from build123d import *

# Parameters (mm, degrees)
SKETCH1_R           = 0.3
SKETCH1_R_2         = 0.6
BOSS_EXTRUDE1_DEPTH = 5


with BuildPart() as part:
    # Sketch1 → Boss-Extrude1 (new body)
    with BuildSketch(Plane(origin=(0, 0, 0), x_dir=(1, 0, 0), z_dir=(0, 1, 0))):
        with BuildLine():
            ThreePointArc((0.1641009, 1.993256355), (0.024548565, 1.994973575), (-0.113883759, 1.977245221))
            Line((-0.113883759, 1.977245221), (-1.25, 1.750241174))
            Line((-1.25, 1.750241174), (-4.183235691, 1.164159973))
            ThreePointArc((-4.183235691, 1.164159973), (-4.514100231, 1.033532975), (-4.77830642, 0.795352694))
            ThreePointArc((-4.77830642, 0.795352694), (-5.05, 0), (-4.77830642, -0.795352694))
            ThreePointArc((-4.77830642, -0.795352694), (-4.514100231, -1.033532975), (-4.183235691, -1.164159973))
            Line((-4.183235691, -1.164159973), (-1.25, -1.750241174))
            Line((-1.25, -1.750241174), (-0.11388376, -1.977245221))
            ThreePointArc((-0.11388376, -1.977245221), (0.024548564, -1.994973575), (0.164100898, -1.993256355))
            ThreePointArc((0.164100898, -1.993256355), (2, -1e-09), (0.1641009, 1.993256355))
        make_face()
        with Locations(Location((-3, 0, 0), (0, 0, 270))):
            Circle(SKETCH1_R, mode=Mode.SUBTRACT)
        with Locations(Location((-1.25, 0, 0), (0, 0, 270))):
            Circle(SKETCH1_R_2, mode=Mode.SUBTRACT)
        with Locations(Location((0.5, 0, 0), (0, 0, 270))):
            Circle(SKETCH1_R, mode=Mode.SUBTRACT)
    extrude(amount=BOSS_EXTRUDE1_DEPTH)


solid = part.part
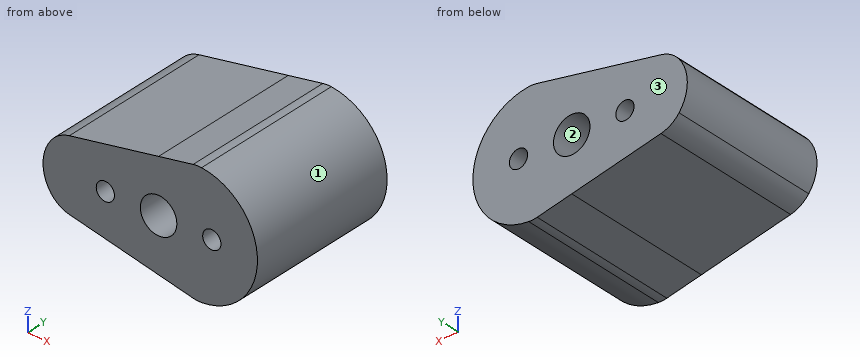
Geometry check sheet. Reference: the model listing, model coordinates, mm. Face numbers are marked on the shaded views. Coordinates: 2 decimals unless noted, no trailing zeros. Order: outer loops, then holes, each group sorted by start corner. A loop starts at its lowest first (then second) coordinate and runs counter-clockwise, first axis right, second up. Notation, with made-up numbers: (84.25, 21) -> (111.25, 21) arc R12 cw to (111.25, 43) -> close; hole circle Ø2 at (87.5, 65.5). An arc over 180 degrees is marked (long way). Use a Markdown table: item, result. Add a question column.
1. Cross-section at A-A (z = 0). Enter the section's corners in (x, y), and give its area (4 significant figures).
2. Material ranges on L1, parallel to Z at x = 0, y = 2.3; L2, parallel to X at y = 0.4, z = -0.35; L3, parallel to Z at x = -2, y = 0.8, recorded low to high.
3. Mould release check, pull along Z, two halves, no side actions. Record for the marked faces 1, 2 and 3: pulls with the +Z half, pulls with the -Z half, needs draft (parallel to the pull), parting line crosses it, or undercut.
4. Cross-section at B-B (x = -3). Enter the section's corners in (y, z).
5. Cross-section at C-C (y = 2.85). Enter the section's corners in (x, z).
6. Go/stop test with a flat-tipped pin: pin 1 Ø2 at (y, z) = (0.5, 1.5) entering from -X. Record where the tip stops, or that it passes through.
7. Cross-section at D-D (z = 0.5). Enter the section's corners in (x, y), and give its area (3 significant figures).
Filled sheet:
| question | item | result |
|---|---|---|
| 1 | outline | (-5.05, 0) -> (-3.3, 0) -> (-3.3, 5) -> (-5.05, 5) -> close; (-2.7, 0) -> (-1.85, 0) -> (-1.85, 5) -> (-2.7, 5) -> close; (-0.65, 0) -> (0.2, 0) -> (0.2, 5) -> (-0.65, 5) -> close; (0.8, 0) -> (2, 0) -> (2, 5) -> (0.8, 5) -> close |
| 1 | area | 23.25 mm2 |
| 2 | L1 | -1.99 to 1.99 |
| 2 | L2 | -5 to -1.74, -0.76 to 1.97 |
| 2 | L3 | -1.6 to 1.6 |
| 3 | face 1 | parting line crosses it |
| 3 | face 2 | undercut |
| 3 | face 3 | needs draft |
| 4 | outline | (0, -1.4) -> (5, -1.4) -> (5, -0.3) -> (0, -0.3) -> close; (0, 0.3) -> (5, 0.3) -> (5, 1.4) -> (0, 1.4) -> close |
| 5 | outline | (-4.78, -0.8) arc R1 ccw to (-4.18, -1.16) -> (-0.11, -1.98) arc R1 ccw to (0.16, -1.99) arc R2 ccw to (0.16, 1.99) arc R1 ccw to (-0.11, 1.98) -> (-4.18, 1.16) arc R1 ccw to (-4.78, 0.8) arc R1.3 ccw to start; hole circle Ø0.6 at (-3, 0); hole circle Ø1.2 at (-1.25, 0); hole circle Ø0.6 at (0.5, 0) |
| 6 | pin 1 | x = -4.95 |
| 7 | outline | (-4.95, 0) -> (-1.58, 0) -> (-1.58, 5) -> (-4.95, 5) -> close; (-0.92, 0) -> (1.94, 0) -> (1.94, 5) -> (-0.92, 5) -> close |
| 7 | area | 31.1 mm2 |
